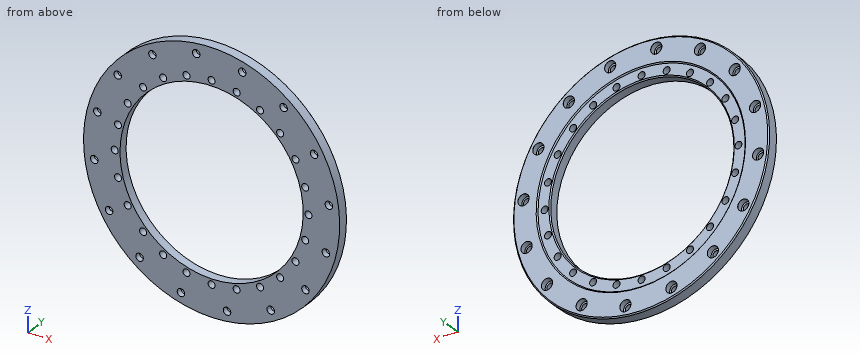
from build123d import *

# Parameters (mm, degrees)
SKETCH2_R          = 6.25
CUT_EXTRUDE3_DEPTH = 20
CIRPATTERN1_COUNT  = 16
CHAMFER1_SIZE      = 2


with BuildPart() as part:
    # Sketch1 → Revolve1 (revolve)
    with BuildSketch(Plane(origin=(0, 0, 0), x_dir=(0, 0, -1), z_dir=(1, 0, 0)), mode=Mode.PRIVATE) as revolve1_sk:
        Polygon((-164.5, 0), (-230, 0), (-230, 20), (-186, 20), (-186, 18), (-164.5, 18), align=None)
    revolve(revolve1_sk.sketch.rotate(Axis((0, 0, 0), (0, 1, 0)), 180), axis=Axis((0, 0, 0), (0, 1, 0)))

    # Sketch2 → Cut-Extrude3 (cut)
    with BuildSketch(Plane(origin=(0, 20, 0), x_dir=(1, 0, 0), z_dir=(0, 1, 0))):
        with Locations(Location((0, 174, 0), (0, 0, 270))):
            Circle(SKETCH2_R)
        with Locations(Location((45.034513848, 168.071093774, 0), (0, 0, 270))):
            Circle(SKETCH2_R)
        with Locations(Location((87, 150.688420258, 0), (0, 0, 270))):
            Circle(SKETCH2_R)
        with Locations(Location((123.036579926, 123.036579926, 0), (0, 0, 270))):
            Circle(SKETCH2_R)
        with Locations(Location((150.688420258, 87, 0), (0, 0, 270))):
            Circle(SKETCH2_R)
        with Locations(Location((168.071093774, 45.034513848, 0), (0, 0, 270))):
            Circle(SKETCH2_R)
        with Locations(Location((174, 0, 0), (0, 0, 270))):
            Circle(SKETCH2_R)
        with Locations(Location((168.071093774, -45.034513848, 0), (0, 0, 270))):
            Circle(SKETCH2_R)
        with Locations(Location((150.688420258, -87, 0), (0, 0, 270))):
            Circle(SKETCH2_R)
        with Locations(Location((123.036579926, -123.036579926, 0), (0, 0, 270))):
            Circle(SKETCH2_R)
        with Locations(Location((87, -150.688420258, 0), (0, 0, 270))):
            Circle(SKETCH2_R)
        with Locations(Location((45.034513848, -168.071093774, 0), (0, 0, 270))):
            Circle(SKETCH2_R)
        with Locations(Location((0, -174, 0), (0, 0, 270))):
            Circle(SKETCH2_R)
        with Locations(Location((-45.034513848, -168.071093774, 0), (0, 0, 270))):
            Circle(SKETCH2_R)
        with Locations(Location((-87, -150.688420258, 0), (0, 0, 270))):
            Circle(SKETCH2_R)
        with Locations(Location((-123.036579926, -123.036579926, 0), (0, 0, 270))):
            Circle(SKETCH2_R)
        with Locations(Location((-150.688420258, -87, 0), (0, 0, 270))):
            Circle(SKETCH2_R)
        with Locations(Location((-168.071093774, -45.034513848, 0), (0, 0, 270))):
            Circle(SKETCH2_R)
        with Locations(Location((-174, 0, 0), (0, 0, 270))):
            Circle(SKETCH2_R)
        with Locations(Location((-168.071093774, 45.034513848, 0), (0, 0, 270))):
            Circle(SKETCH2_R)
        with Locations(Location((-150.688420258, 87, 0), (0, 0, 270))):
            Circle(SKETCH2_R)
        with Locations(Location((-123.036579926, 123.036579926, 0), (0, 0, 270))):
            Circle(SKETCH2_R)
        with Locations(Location((-87, 150.688420258, 0), (0, 0, 270))):
            Circle(SKETCH2_R)
        with Locations(Location((-45.034513848, 168.071093774, 0), (0, 0, 270))):
            Circle(SKETCH2_R)
    extrude(amount=-CUT_EXTRUDE3_DEPTH, mode=Mode.SUBTRACT)

    # Sketch7 → CBORE for M12 SHCS1 (revolve, cut)
    with BuildSketch(Plane(origin=(27.736815847, 20, -210.682033042), x_dir=(0, 0, 1), z_dir=(1, 0, 0))):
        Polygon((0, 0), (0, 20), (6.75, 20), (6.75, 10), (10, 10), (10, 0.025), (10.025, 0), align=None)
    cbore_for_m12_shcs1 = revolve(axis=Axis((27.736815847, 26.35, -210.682033042), (0, -1, 0)), mode=Mode.SUBTRACT)

    # CirPattern1: CBORE for M12 SHCS1 ×16 about axis
    cirpattern1_axis = Axis((0, 0, 0), (0, 1, 0))
    for i in range(1, CIRPATTERN1_COUNT):
        add(cbore_for_m12_shcs1.rotate(cirpattern1_axis, i * 360 / CIRPATTERN1_COUNT), mode=Mode.SUBTRACT)

    # Chamfer1
    chamfer1_edges = [part.edges().sort_by_distance(p)[0] for p in [
        (0, 20, 186),
        (0, 20, 230),
        (0, 18, 164.5),
    ]]
    chamfer(chamfer1_edges, length=CHAMFER1_SIZE - 0.0001)  # a hair under: the kernel refuses the full size


solid = part.part
The listing builds one solid part. Answer for the finished solid, in the listing's coordinates (mm). Coordinates: 2 decimals unless noted, no trailing zeros. Answer in a Markdown table with one row per item. Add a question column.
1. Consider line 1 (Z direction, x = 1, y = 3.5); line 2 (Z direction, x = 31, y = 6.25); line 3 (X direction, y = 13, z = -24). Determine where each line is inside the solid, lowest interval first. Write a range as [from, to].
2. Flat-ended cylindrical pins translate along their axes: P1, Ø11, axis at x = -210.68, z = -27.74, coming from the +Y side; P2, Ø1, axis at x = 27, y = 16.5, coming from the -Z side; P3, Ø15.5, axis at x = 184.03, z = 106.25, coming from the +Y side; P4, Ø12, axis at y = 9, z = -45.5, coming from the -X side. Find the tip coordinate at first contact, or state that the pin passes through.
3. The part is cut by section A-A, the plane x = 0. Count the separate pieces of the cut face and the enclosed holes in it, then the cut area to 3 significant figures.
Answer below:
| question | item | result |
|---|---|---|
| 1 | line 1 | [-230, -180.17], [-167.83, -164.5], [164.5, 167.83], [180.17, 230] |
| 1 | line 2 | [-227.9, -216.59], [-204.77, -161.55], [161.55, 227.9] |
| 1 | line 3 | [-228.74, -219.96], [-201.41, -162.74], [162.74, 228.74] |
| 2 | P1 | through |
| 2 | P2 | z = -228.47 |
| 2 | P3 | y = 10 |
| 2 | P4 | x = -226.58 |
| 3 | separate pieces | 4 |
| 3 | enclosed holes | 0 |
| 3 | area | 2,070 mm2 |
